Autodesk Fusion 360 part; units mm, degrees
sketch "Onderkant" plane through (0, 0, 0) normal (0, 0, 1) x (1, 0, 0)
  line L0 (250, 150) -> (-250, 150)
  line L1 (-250, 150) -> (-250, -150)
  line L2 (-250, -150) -> (250, -150)
  line L3 (250, -150) -> (250, 150)
  line L4 (250, 150) -> (-250, -150) construction
  line L5 (-250, 150) -> (250, -150) construction
  dimension "d29" = 500
  dimension "d30" = 300
extrude "Extrude7" add sketch "Onderkant" along normal blind 6
sketch "Zijkanten" plane through (0, 0, 6) normal (0, 0, 1) x (-1, 0, 0)
  line L0 (-250, 150) -> (-250, -150)
  line L1 (-250, -150) -> (250, -150)
  line L2 (250, -150) -> (250, 150)
  line L3 (250, 150) -> (-250, 150)
  line L4 (-247, 147) -> (247, 147)
  line L5 (247, 147) -> (247, -147)
  line L6 (247, -147) -> (-247, -147)
  line L7 (-247, -147) -> (-247, 147)
  line L8 (-247, 147) -> (247, -147) construction
  line L9 (247, 147) -> (-247, -147) construction
  dimension "d33" = 494
  dimension "d34" = 294
extrude "Extrude8" add sketch "Zijkanten" along normal blind 300
sketch "Bovenkant" plane through (0, 0, 306) normal (0, 0, 1) x (-1, 0, 0)
  line L0 (247, -147) -> (-247, -147)
  line L1 (-247, -147) -> (-247, 147)
  line L2 (-247, 147) -> (247, 147)
  line L3 (247, 147) -> (247, -147)
  line L4 (250, 150) -> (-250, 150)
  line L5 (-250, 150) -> (-250, -150)
  line L6 (-250, -150) -> (250, -150)
  line L7 (250, -150) -> (250, 150)
  line L8 (-250, 150) -> (250, 150)
  line L9 (250, 150) -> (250, -150)
  line L10 (250, -150) -> (-250, -150)
  line L11 (-250, -150) -> (-250, 150)
  line L12 (-250, 150) -> (250, -150) construction
  line L13 (250, 150) -> (-250, -150) construction
  dimension "d37" = 500
  dimension "d38" = 300
extrude "Extrude9" add sketch "Bovenkant" against normal blind 6 contours L0 L1 L2 L3
sketch "Deur" plane through (0, -150, 0) normal (0, -1, 0) x (1, 0, 0)
  line L0 (-250, 0) -> (250, 0)
  line L1 (250, 0) -> (250, 306)
  line L2 (250, 306) -> (-250, 306)
  line L3 (-250, 306) -> (-250, 0)
  line L4 (200, 6) -> (-100, 6)
  line L5 (-100, 6) -> (-100, 206)
  line L6 (-100, 206) -> (200, 206)
  line L7 (200, 206) -> (200, 6)
  dimension "d42" = 300
  dimension "d43" = 200
extrude "Extrude10" cut sketch "Deur" against normal blind 6 contours L4 L5 L6 L7
sketch "Gat kabel" plane through (0, 150, 0) normal (0, 1, 0) x (-1, 0, 0)
  line L0 (-250, 0) -> (250, 0)
  line L1 (250, 0) -> (250, 306)
  line L2 (250, 306) -> (-250, 306)
  line L3 (-250, 306) -> (-250, 0)
  line L4 (240, 10) -> (220, 10)
  line L5 (220, 10) -> (220, 30)
  line L6 (220, 30) -> (240, 30)
  line L7 (240, 30) -> (240, 10)
  circle A0 centre (230, 20) radius 6
  dimension "d46" = 12
extrude "Extrude11" cut sketch "Gat kabel" against normal blind 6 contours A0
sketch "Gat scanner" plane through (0, -150, 0) normal (0, -1, 0) x (1, 0, 0)
  line L0 (-100, 6) -> (-100, 206)
  line L1 (-100, 206) -> (200, 206)
  line L2 (200, 206) -> (200, 6)
  line L3 (200, 6) -> (-100, 6)
  line L4 (-250, 0) -> (250, 0)
  line L5 (250, 0) -> (250, 306)
  line L6 (250, 306) -> (-250, 306)
  line L7 (-250, 306) -> (-250, 0)
  line L8 (67.5, 268.5) -> (32.5, 268.5)
  line L9 (32.5, 268.5) -> (32.5, 243.5)
  line L10 (32.5, 243.5) -> (67.5, 243.5)
  line L11 (67.5, 243.5) -> (67.5, 268.5)
  line L12 (67.5, 268.5) -> (32.5, 243.5) construction
  line L13 (32.5, 268.5) -> (67.5, 243.5) construction
  point P0 (50, 256)
  dimension "d51" = 35
  dimension "d52" = 25
extrude "Extrude12" cut sketch "Gat scanner" against normal blind 6 contours L8 L9 L10 L11
equation "lengte = 500 mm"
equation "breedte = 300 mm"
equation "hoogte = 300 mm"
equation "dikte_plaat = 6 mm"
equation "breedte_deur = 300 mm"
equation "hoogte_deur = 200 mm"
equation "d29 = lengte"
equation "d30 = breedte"
equation "d31 = dikte_plaat"
equation "d33 = lengte - dikte_plaat"
equation "d34 = breedte - dikte_plaat"
equation "d35 = hoogte"
equation "d37 = lengte"
equation "d38 = breedte"
equation "d42 = breedte_deur"
equation "d43 = hoogte_deur"
equation "breedte_scanner = 35 mm"
equation "hoogte_scanner = 25 mm"
equation "d51 = breedte_scanner"
equation "d52 = hoogte_scanner"
Work out the finished part from the listing and answer in its coordinate system (mm). A direction names the side the tool comes from. Round coordinates to 2 decimals unless told otherwise and drop trailing zeros. Loops run counter-clockwise (first coordinate to the right, second up) from the corner with the lowest first, then second, coordinate; pieces in that order, holes last.
(1) Find the intervals of material crossed by L1, parallel to Z at x = -230, y = 149; L2, parallel to X at y = 129.5, z = 139.5; L3, parallel to Z at x = 30.5, y = 0.5, in increasing order.
Computed values:
L1: z = 0 to 14, 26 to 306
L2: x = -250 to -247, 247 to 250
L3: z = 0 to 6, 300 to 306
(2) The part is cut by section A-A, the plane y = -38. Give the vertices of the cut face in (x, z), and give its area (3 significant figures).
Computed values:
outline: (-250, 0) - (250, 0) - (250, 306) - (-250, 306) - close; hole (-247, 6) - (247, 6) - (247, 300) - (-247, 300) - close
area: 7,760 mm2
(3) The part is cut by section D-D, the plane z = 164. Give the vertices of the cut face in (x, y), and give its area (3 significant figures).
Computed values:
outline: (-250, -150) - (-100, -150) - (-100, -147) - (-247, -147) - (-247, 147) - (247, 147) - (247, -147) - (200, -147) - (200, -150) - (250, -150) - (250, 150) - (-250, 150) - close
area: 3,860 mm2
(4) The part is cut by section B-B, the plane x = -230. Give the vertices of the cut face in (y, z), and give its area (3 significant figures).
Computed values:
outline: (-150, 0) - (150, 0) - (150, 14) - (147, 14) - (147, 6) - (-147, 6) - (-147, 300) - (147, 300) - (147, 26) - (150, 26) - (150, 306) - (-150, 306) - close
area: 5,330 mm2
(5) The part is cut by section C-C, the plane z = 20. Give the vertices of the cut face in (x, y), and give its area (3 significant figures).
Computed values:
outline: (-250, -150) - (-100, -150) - (-100, -147) - (-247, -147) - (-247, 147) - (-236, 147) - (-236, 150) - (-250, 150) - close; (-224, 147) - (247, 147) - (247, -147) - (200, -147) - (200, -150) - (250, -150) - (250, 150) - (-224, 150) - close
area: 3,830 mm2
(6) The mould has two halves that part along Y. Classify faces 1 (the flat face through (-250, 2, 151)), 2 (the flat face through (-247, -2, 151)), 3 (the flat face through (-59, -150, 219)): pulls with the +Y half, pulls with the -Y half, needs draft (parallel to the pull), parting line crosses it, or undercut.
Computed values:
face 1: needs draft
face 2: undercut
face 3: pulls with the -Y half
(7) For faces 4 (the cylindrical face through (-235.723, 148.521, 21.802)), 5 (the flat face through (3, -4, 6)), 6 (the flat face through (3, -2, 306)), determine the directions among +Z, -Z, +X, -X, +Y, -Y from which every point of the face is accessible in a straight line to the end or side of a thin tool.
Computed values:
face 4: +Y
face 5: none
face 6: +Z, +X, -X, +Y, -Y
(8) This flat-tipped pin is pushed along its axis until it touches: P1, Ø12, axis at x = 36.5, z = 126, coming from the -Y side. Where does it stop, or does it pass through?
Computed values:
P1: stops at y = 147
